Drawing for the job (mm, zero at the part's lowest x, y, z). A direction names the side the tool comes from. Give positions to 0.01 mm unless a question says otherwise; leave off trailing zeros. Loops run counter-clockwise (first coordinate to the right, second up) from the corner with the lowest first, then second, coordinate; pieces in that order, holes last.
1) Band-saw the part on A-A on z = 26.5. List the corners of the cut face in (x, y).
2) Two-plate mould, pull along X, no slides. Class the marked faces 1, 2 and 3: +X half, -X half, draft (parallel to the pull), parting line (faces both ways), or undercut.
3) Band-saw the part on D-D on z = 136. List the corners of the cut face in (x, y).
4) Band-saw the part on C-C on y = 35.5. List the corners of the cut face in (x, z), then the cut area to 3 significant figures.
5) Wall check: line 1 (X direction, y = 42, z = 88.5); line 2 (Y direction, x = 107, z = 3); line 3 (Z direction, x = 160, y = 24). Give the ranges that are in metal, low to high.
6) 3-axis set-ups, long thin cutter, end or side, ignore diameter. For the marked faces 4 and 5: which of +Z, -Z, +X, -X, +Y, -Y reach the whole face in a straight line?
7) Band-saw the part on B-B on x = 107. List the corners of the cut face in (y, z), then the cut area to 3 significant figures.
8) Flat gauge pins, fed straight in: P1, Ø10, axis at x = 59.5, y = 174, coming from the +Z side; P2, Ø8, axis at x = 103.5, y = 114.5, coming from the -Z side. Where does each tip first touch, or does it go through?
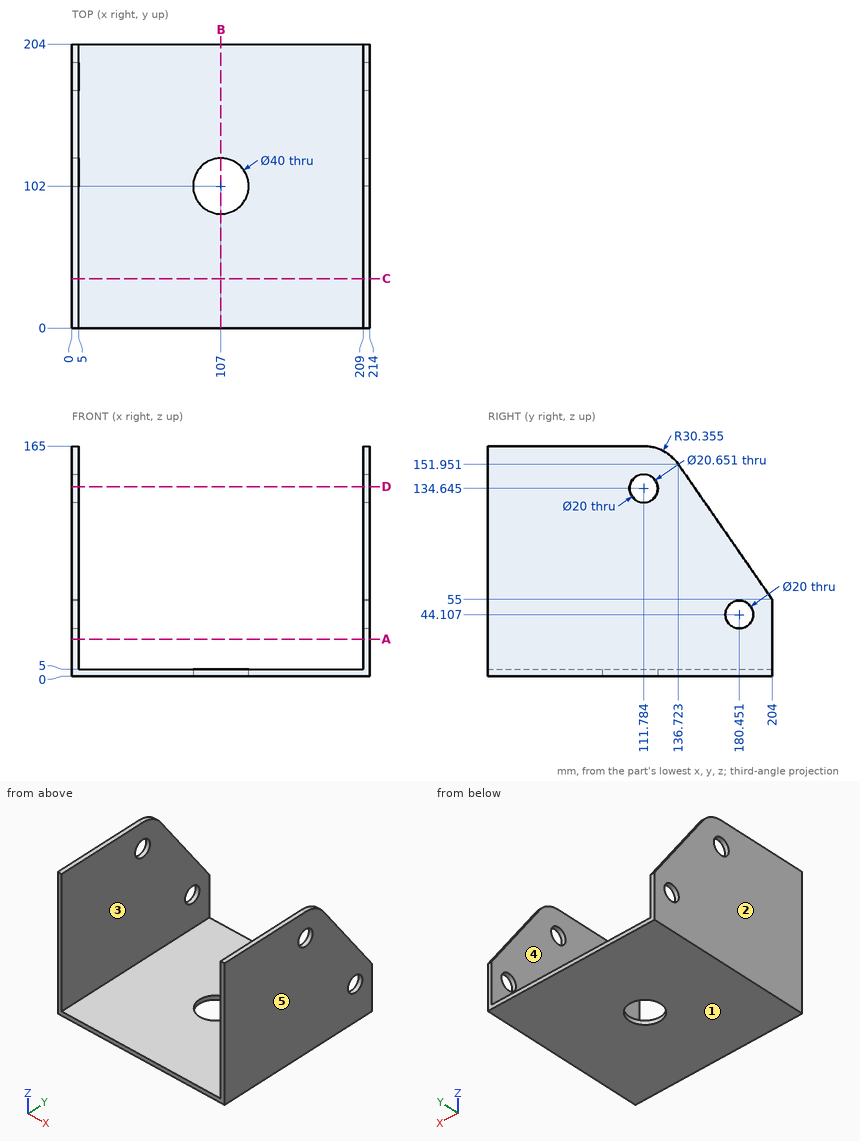
Findings below:
1. outline: (0, 0) - (5, 0) - (5, 204) - (0, 204) - close; (209, 0) - (214, 0) - (214, 204) - (209, 204) - close
2. face 1: draft
2. face 2: -X half
2. face 3: undercut
3. outline: (0, 0) - (5, 0) - (5, 101.55) - (0, 101.55) - close; (0, 122.02) - (5, 122.02) - (5, 147.79) - (0, 147.79) - close; (209, 0) - (214, 0) - (214, 101.88) - (209, 101.88) - close; (209, 121.69) - (214, 121.69) - (214, 147.79) - (209, 147.79) - close
4. outline: (0, 0) - (214, 0) - (214, 165) - (209, 165) - (209, 5) - (5, 5) - (5, 165) - (0, 165) - close
4. area: 2,670 mm2
5. line 1: x = 0 to 5, 209 to 214
5. line 2: y = 0 to 82, 122 to 204
5. line 3: z = 0 to 5
6. face 4: +Z, +Y, -Y
6. face 5: +Z, -Z, +X, +Y, -Y
7. outline: (0, 0) - (82, 0) - (82, 5) - (0, 5) - close; (122, 0) - (204, 0) - (204, 5) - (122, 5) - close
7. area: 820 mm2
8. P1: stops at z = 5
8. P2: passes through
